from build123d import *

# Parameters (mm, degrees)
SKETCH_1_W          = 91
SKETCH_1_H          = 74
SKETCH_1_R          = 1.6
EXTRUDE_1_DEPTH     = 3
SKETCH_2_R          = 30
SKETCH_2_R_2        = 1.6
CUT_EXTRUDE_1_DEPTH = 10
SKETCH_3_W          = 91
SKETCH_3_H          = 6
CUT_EXTRUDE_2_DEPTH = 10
SKETCH_4_W          = 91
SKETCH_4_H          = 8.5
SKETCH_4_H_2        = 14.5
EXTRUDE_2_DEPTH     = 3
SKETCH_5_W          = 91
SKETCH_5_H          = 6
CUT_EXTRUDE_3_DEPTH = 3
FILLET_4_R          = 25


with BuildPart() as part:
    # 草图1 → 凸台-拉伸1 (new body)
    with BuildSketch(Plane.XY):
        Rectangle(SKETCH_1_W, SKETCH_1_H)
        with Locations((36, -25)):
            Circle(SKETCH_1_R, mode=Mode.SUBTRACT)
        with Locations((36, 25)):
            Circle(SKETCH_1_R, mode=Mode.SUBTRACT)
        with Locations(Location((-36, 25, 0), (0, 0, 180))):
            Circle(SKETCH_1_R, mode=Mode.SUBTRACT)
        with Locations(Location((-36, -25, 0), (0, 0, 180))):
            Circle(SKETCH_1_R, mode=Mode.SUBTRACT)
    extrude(amount=EXTRUDE_1_DEPTH)

    # 草图2 → 切除-拉伸1 (cut)
    with BuildSketch(Plane.XY.offset(3)):
        with Locations((0, -3)):
            Circle(SKETCH_2_R)
        with Locations((24.748737342, -27.748737342)):
            Circle(SKETCH_2_R_2)
        with Locations((24.748737342, 21.748737342)):
            Circle(SKETCH_2_R_2)
        with Locations((-24.748737342, -27.748737342)):
            Circle(SKETCH_2_R_2)
        with Locations((-24.748737342, 21.748737342)):
            Circle(SKETCH_2_R_2)
    extrude(amount=-CUT_EXTRUDE_1_DEPTH, mode=Mode.SUBTRACT)

    # 草图3 → 切除-拉伸2 (cut)
    with BuildSketch(Plane.XY.offset(3)):
        with Locations((0, 34)):
            Rectangle(SKETCH_3_W, SKETCH_3_H)
    extrude(amount=-CUT_EXTRUDE_2_DEPTH, mode=Mode.SUBTRACT)

    # 草图4 → 凸台-拉伸2 (add)
    with BuildSketch(Plane.XY.offset(3)):
        with Locations((0, -41.25)):
            Rectangle(SKETCH_4_W, SKETCH_4_H)
        with Locations((0, 38.25)):
            Rectangle(SKETCH_4_W, SKETCH_4_H_2)
    extrude(amount=-EXTRUDE_2_DEPTH)

    # 草图5 → 切除-拉伸3 (cut)
    with BuildSketch(Plane.XY.offset(3)):
        with Locations((0, 42.5)):
            Rectangle(SKETCH_5_W, SKETCH_5_H)
    extrude(amount=-CUT_EXTRUDE_3_DEPTH, mode=Mode.SUBTRACT)

    # 圆角4
    fillet_4_edges = [part.edges().sort_by_distance(p)[0] for p in [
        (-45.5, 39.5, 1.5),
        (45.5, 39.5, 1.5),
        (-45.5, -45.5, 1.5),
        (45.5, -45.5, 1.5),
    ]]
    fillet(fillet_4_edges, radius=FILLET_4_R)


solid = part.part
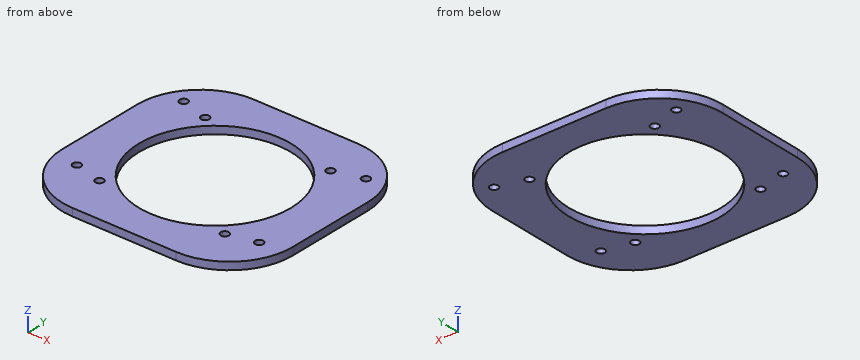
Geometry: final body of the model. Coordinates: model frame, mm. Give positions to 0.01 mm unless a question says otherwise; leave off trailing zeros. Write each loop counter-clockwise with the first axis right and the second up, starting at its lowest first coordinate (ties: lowest second). Pieces come first, ordered by that corner, then holes. Notation, with made-up numbers: (-33, -33.75) - (24, -33.75) arc R25 cw to (24, -1.75) - close; hole circle Ø3 at (19, -9.75). An arc over 180 degrees is marked (long way). Return JSON: item names as keys, results as strings. Group by question number.
1) Section C-C on z = 2.2. State how many separate pieces and enclosed holes the cut face has, plus the area to 3 significant figures.
2) Line query: line 1 (Y direction, x = 36, z = 0.6); line 2 (X direction, y = 24.5, z = 1.2); line 3 (Y direction, x = 0, z = 1.85). Output: solid intervals per line, ascending.
3) First-contact query: P1, Ø1.5, axis at x = -25, z = 1.5, coming from the -Y side. Flat tip, straight axial feed; report the tip coordinate or a pass-through.
4) Section D-D on x = 36. Return the cut outline in (y, z), plus the area to 3 significant figures.
5) Section A-A on x = 0. Return the cut outline in (y, z), plus the area to 3 significant figures.
6) Section B-B on y = -13. Return the cut outline in (x, z), plus the area to 3 significant figures.
Filled in:
{
 "1": {"separate pieces": "1", "enclosed holes": "9", "area": "4,310 mm^2"},
 "2": {"line 1": "y = -40.12 to -26.6, -23.4 to 23.4, 26.6 to 34.12", "line 2": "x = -43.41 to -37.52, -34.48 to -11.99, 11.99 to 34.48, 37.52 to 43.41", "line 3": "y = -45.5 to -33, 27 to 39.5"},
 "3": {"P1": "stops at y = -45.22"},
 "4": {"outline": "(-40.12, 0) - (-26.6, 0) - (-26.6, 3) - (-40.12, 3) - close; (-23.4, 0) - (23.4, 0) - (23.4, 3) - (-23.4, 3) - close; (26.6, 0) - (34.12, 0) - (34.12, 3) - (26.6, 3) - close", "area": "203 mm^2"},
 "5": {"outline": "(-45.5, 0) - (-33, 0) - (-33, 3) - (-45.5, 3) - close; (27, 0) - (39.5, 0) - (39.5, 3) - (27, 3) - close", "area": "75.0 mm^2"},
 "6": {"outline": "(-45.5, 0) - (-28.28, 0) - (-28.28, 3) - (-45.5, 3) - close; (28.28, 0) - (45.5, 0) - (45.5, 3) - (28.28, 3) - close", "area": "103 mm^2"}
}
